Input: part model. Units: mm. Frame: model coordinates. A direction names the side the tool comes from. Coordinates: 2 decimals unless noted, no trailing zeros. Write each loop counter-clockwise with the first axis right and the second up, starting at its lowest first coordinate (ties: lowest second). Pieces come first, ordered by that corner, then holes. Notation, with made-up numbers: (0, -37) - (23, -37) arc R31 ccw to (23, -13) - close; hole circle Ø2 at (-16, 13.5). An arc over 180 degrees is marked (long way). Use a Markdown table: item, result. Add a question column.
Q1. Section query D-D (x = 3). Return the cut outline in (y, z), then the cut area to 3 significant figures.
Q2. Section query A-A (x = 0). Return the cut outline in (y, z).
Q3. Mould query, pull axis X, two halves, no side actions, for faces 1 (the face through (0, 11, 14)), 2 (the face through (10, 7, 1)), 3 (the face through (-1.5, 11, 9)). Classes: released by +X, released by -X, zero draft, split by the parting line, or undercut.
Q4. Material intervals for probe 1 along Y at (x, z) = (0, 0.55); probe 2 along X at (y, z) = (2, 0.6); probe 3 along Z at (x, y) = (-1, 10.5), sorted ascending. Write a range as from..to.
Q5. Pin query (flat end, axial travel): P1, Ø6, axis at x = -3.5, y = 3, coming from the +Z side; P2, Ø3, axis at x = 5, z = 6.5, coming from the -Y side; P3, Ø3, axis at y = 7, z = 12.5, coming from the -X side. Return the tip coordinate at first contact, or that it passes through.
Q6. Section query C-C (z = 10). Return the cut outline in (x, y).
Q7. Set-up query: faces 4 (the face through (-10, 7, 1)), 5 (the face through (0, 4, 2)), 6 (the face through (0, 11, 7)). Return all of +Z, -Z, +X, -X, +Y, -Y with unobstructed straight access to the full face (end or side cutting, diameter ignored); none if empty.
Q8. Section query B-B (y = 2). Return the cut outline in (x, z).
Autodesk Fusion 360 part; units mm, degrees
sketch "Szkic1" plane through (0, 0, 0) normal (0, 0, 1) x (1, 0, 0)
  line L0 (-10, 10) -> (10, 10)
  line L1 (10, 10) -> (10, -5)
  line L2 (10, -5) -> (-10, -5)
  line L3 (-10, -5) -> (-10, 10)
  circle A0 centre (0, 2) radius 1
  dimension "d1" = 15
  dimension "d10" = 2
extrude "Wyciągnięcie proste1" add sketch "Szkic1" along normal blind 2 contours L0 L1 L2 L3 | A0
sketch "Szkic2" plane through (0, 10, 0) normal (0, 1, 0) x (-1, 0, 0)
  line L0 (-10, 0) -> (10, 0)
  line L1 (10, 0) -> (10, 2)
  line L2 (10, 2) -> (-10, 2)
  line L3 (-10, 2) -> (-10, 0)
  line L4 (-10, 0) -> (10, 0)
  line L5 (10, 0) -> (10, 14)
  line L6 (10, 14) -> (-10, 14)
  line L7 (-10, 14) -> (-10, 0)
  line L8 (1.5, 11) -> (-1.5, 11)
  line L9 (-1.5, 11) -> (-1.5, 7)
  line L10 (-1.5, 7) -> (1.5, 7)
  line L11 (1.5, 7) -> (1.5, 11)
  dimension "d4" = 8.5
  dimension "d5" = 3
  dimension "d6" = 20
  dimension "d7" = 3
extrude "Wyciągnięcie proste2" add sketch "Szkic2" along normal blind 2
extrude "Wyciągnięcie proste3" cut sketch "Szkic1" along normal blind 3 contours A0
Values follow:
| question | item | result |
|---|---|---|
| 1 | outline | (-5, 0) - (12, 0) - (12, 14) - (10, 14) - (10, 2) - (-5, 2) - close |
| 1 | area | 58.0 mm2 |
| 2 | outline | (-5, 0) - (1, 0) - (1, 2) - (-5, 2) - close; (3, 0) - (12, 0) - (12, 7) - (10, 7) - (10, 2) - (3, 2) - close; (10, 11) - (12, 11) - (12, 14) - (10, 14) - close |
| 3 | face 1 | zero draft |
| 3 | face 2 | released by +X |
| 3 | face 3 | undercut |
| 4 | probe 1 | -5..1, 3..12 |
| 4 | probe 2 | -10..-1, 1..10 |
| 4 | probe 3 | 0..7, 11..14 |
| 5 | P1 | z = 2 |
| 5 | P2 | y = 10 |
| 5 | P3 | through |
| 6 | outline | (-10, 10) - (-1.5, 10) - (-1.5, 12) - (-10, 12) - close; (1.5, 10) - (10, 10) - (10, 12) - (1.5, 12) - close |
| 7 | face 4 | +Z, -Z, -X, +Y, -Y |
| 7 | face 5 | +Z, +X, -X, -Y |
| 7 | face 6 | +Y, -Y |
| 8 | outline | (-10, 0) - (-1, 0) - (-1, 2) - (-10, 2) - close; (1, 0) - (10, 0) - (10, 2) - (1, 2) - close |
